The listing builds one solid part. Answer for the finished solid, in the listing's coordinates (mm). A direction names the side the tool comes from. Coordinates: 2 decimals unless noted, no trailing zeros. Write each loop counter-clockwise with the first axis right and the second up, starting at its lowest first coordinate (ties: lowest second). Pieces come first, ordered by that corner, then holes.
Autodesk Inventor part; units mm, degrees
ref_plane "YZ Plane" through (0, 0, 0) normal (1, 0, 0) x (0, 1, 0)
ref_plane "XZ Plane" through (0, 0, 0) normal (0, 1, 0) x (-1, 0, 0)
ref_plane "XY Plane" through (0, 0, 0) normal (0, 0, 1) x (1, 0, 0)
sketch "Sketch1" plane through (0, 0, 0) normal (0, 1, 0) x (-1, 0, 0)
  line L0 (0, 0) -> (-4.5, 0)
  line L1 (-4.5, 0) -> (-4.5, -14.5)
  line L2 (-4.5, -14.5) -> (0, -14.5)
  line L3 (0, -14.5) -> (0, 0)
  circle A0 centre (-2.25, -7.25) radius 1.5
  line L4 (-1.65, -13.75) -> (-1.65, -9)
  line L5 (-1.65, -5.5) -> (-1.65, -0.75)
  line L6 (-2.85, -13.75) -> (-2.85, -9)
  line L7 (-2.85, -5.5) -> (-2.85, -0.75)
  line L8 (-1.65, -0.75) -> (-2.85, -0.75)
  line L9 (-1.65, -13.75) -> (-2.85, -13.75)
  line L10 (-1.65, -11.7) -> (-2.85, -11.7)
  line L11 (-1.65, -2.8) -> (-2.85, -2.8)
  circle A1 centre (-2.25, -7.25) radius 1.85
  dimension "d0" = 4.5
  dimension "d2" = 3
  dimension "d9" = 3.7
  dimension "d32" = 7.25
  dimension "d33" = 7.25
extrude "Extrusion1" add sketch "Sketch1" against normal blind 1.6 contours L3 L2 L1 L0 | A0 | L9 L6 L10 L4 | L10 L6 A1 L4 | A1 | L7 L11 L5 A1 | L7 L8 L5 L11
extrude "Extrusion2" add sketch "Sketch1" along normal blind 2 contours L9 L6 L10 L4 | L7 L8 L5 L11
extrude "Extrusion3" add sketch "Sketch1" along normal blind 5 contours L10 L6 A1 L4 | A1 | L7 L11 L5 A1
fillet "Fillet1" radius 0.2 4 edges at (2.25, 5, -2.8) (2.25, 5, -11.7) (2.25, 2, -0.75) (2.25, 2, -13.75)
thread "Thread1"
sketch "Sketch2" plane through (2.25, 0, -7.25) normal (0, 1, 0) x (1, 0, 0)
  circle A0 centre (0, 0) radius 1.5
  point P0 (-2.25, -7.25)
extrude "Extrusion4" cut sketch "Sketch2" against normal blind 10
properties part number "fixação do pino" material "Aluminum 6061-AHC"
Q1. The part is cut by section B-B, the plane x = 2.25. Write down the section's boundary in (y, z), then the cut area to 3 significant figures.
Answers below:
outline: (-1.6, -14.5) - (0, -14.5) - (0, -13.75) - (1.8, -13.75) arc R0.2 ccw to (2, -13.55) - (2, -11.7) - (4.8, -11.7) arc R0.2 ccw to (5, -11.5) - (5, -8.75) - (-1.6, -8.75) - close; (-1.6, -5.75) - (5, -5.75) - (5, -3) arc R0.2 ccw to (4.8, -2.8) - (2, -2.8) - (2, -0.95) arc R0.2 ccw to (1.8, -0.75) - (0, -0.75) - (0, 0) - (-1.6, 0) - close
area: 56.1 mm2
Q2. The part is cut by section A-A, the plane z = -7.25. Write down the section's boundary in (x, y).
Answers below:
outline: (0, -1.6) - (0.75, -1.6) - (0.75, 5) - (0.4, 5) - (0.4, 0) - (0, 0) - close; (3.75, -1.6) - (4.5, -1.6) - (4.5, 0) - (4.1, 0) - (4.1, 5) - (3.75, 5) - close
Q3. The part is cut by section D-D, the plane z = -4.25. Write down the section's boundary in (x, y).
Answers below:
outline: (0, -1.6) - (4.5, -1.6) - (4.5, 0) - (2.85, 0) - (2.85, 5) - (1.65, 5) - (1.65, 0) - (0, 0) - close
Q4. The part is cut by section C-C, the plane y = 2.5. Write down the section's boundary in (x, z), then the cut area to 3 significant figures.
Answers below:
outline: (1.65, -11.7) - (2.85, -11.7) - (2.85, -9) arc R1.85 ccw to (2.85, -5.5) - (2.85, -2.8) - (1.65, -2.8) - (1.65, -5.5) arc R1.85 ccw to (1.65, -9) - close; hole circle Ø3 at (2.25, -7.25)
area: 10.0 mm2
Q5. Which of the six approach directions +Z, -Z, +X, -X, +Y, -Y give full straight-line access (tool end or side, diameter ignored) to faces 1 (the face through (1.65, 2, -4)), 2 (the face through (2.85, 2, -4)), 3 (the face through (2, 1, -13.75)), 4 (the face through (2, 3, -2.8))?
Answers below:
face 1: +Z, -X, +Y
face 2: +Z, +X, +Y
face 3: -Z, +X, -X, +Y
face 4: +Z, +X, -X, +Y
Q6. Given pin 1 (1 mm diameter, centred on x = 2.5, z = -13, fed in from +Y); pin 2 (1.3 mm diameter, centred on x = 2.5, y = 1, fed in from +Z); pin 3 (0.6 mm diameter, centred on x = 2.5, y = 3, fed in from +Z); pin 4 (2.5 mm diameter, centred on x = 2.25, z = -7.25, fed in from -Y), each flat-ended and moving along its own axis, determine where each tip first touches the part or whether it passes through.
Answers below:
pin 1: stops at y = 2
pin 2: stops at z = -0.75
pin 3: stops at z = -2.8
pin 4: passes through
Q7. Find the intervals of material crossed by probe 1 along Z at (x, y) = (2.25, -0.7); probe 2 along X at (y, z) = (-0.55, -7.25); probe 3 along Z at (x, y) = (2.15, 2.25), in increasing order.
Answers below:
probe 1: z = -14.5 to -8.75, -5.75 to 0
probe 2: x = 0 to 0.75, 3.75 to 4.5
probe 3: z = -11.7 to -8.75, -5.75 to -2.8
